Here's how the part is built. I have some questions about the finished solid (model axes, mm). A direction names the side the tool comes from. Give positions to 0.01 mm unless a question says otherwise; leave off trailing zeros. Loops run counter-clockwise (first coordinate to the right, second up) from the corner with the lowest first, then second, coordinate; pieces in that order, holes last. Notation, with made-up numbers: M 7,-28 L 43,-28 A10 cw 43,-13 Z; hole C 21,28.5 d9. An arc over 180 degrees is marked long. Write item = value, one per line. Start each with the question number.
```python
from build123d import *


with BuildPart() as part:
    # Sketch1 → Revolve1 (revolve)
    with BuildSketch(Plane.XY):
        with BuildLine():
            Line((0, 16.845299462), (2, 18))
            Line((2, 18), (10, 18))
            Line((10, 18), (10, 22.5))
            Line((10, 22.5), (37, 22.5))
            ThreePointArc((37, 22.5), (39.121320344, 21.621320344), (40, 19.5))
            Line((40, 19.5), (40, 15))
            Line((40, 15), (12.772080403, 14.049180096))
            ThreePointArc((12.772080403, 14.049180096), (12.22452816, 13.805394131), (12, 13.249667434))
            Line((12, 13.249667434), (12, 5.1))
            Line((12, 5.1), (0, 5.1))
            Line((0, 5.1), (0, 16.845299462))
        make_face()
    revolve(axis=Axis((0, 0, 0), (1, 0, 0)))


solid = part.part
```
Q1. If we section it at D-D, the plane x = 8: List the corners of the cut face in (y, z) for me.
Q2. We'd pull the mould along Y, two halves only. Please class faces 4 (the cylindrical face through (5.9, 2.4, -4.5)), 5 (the flat face through (10, 10.1, 15.1)), 6 (the conical face through (0.13, 16.14, 5.08)): pulls with the +Y half, pulls with the -Y half, needs draft (parallel to the pull), parting line crosses it, or undercut.
Q3. Will these pins go through, and if not, where does the flat tip stop? pin 1 (8 mm diameter, centred on y = 6, z = 2.5, fed in from +X); pin 2 (3 mm diameter, centred on y = 1, z = -1.5, fed in from +X); pin 3 (1 mm diameter, centred on x = 23.5, z = 6.5, fed in from +Y); pin 4 (12 mm diameter, centred on x = 30.5, y = -18, fed in from -Z).
Q4. On a 3-axis mill with a long thin cutter (end or side, diameter ignored), from which of +Z, -Z, +X, -X, +Y, -Y can I reach the whole of each face in a straight line? I mean faces 1 (the flat face through (12, 0, -6)), 2 (the cylindrical face through (6.056, -2.343, 17.847)), 3 (the cylindrical face through (23.689, 10.382, -19.961)). Say none if no direction works.
Q5. If I drill on line 1 along Z through (x, y) = (3, 0); line 2 along Y through (x, z) = (20, -4); line 3 along Y through (x, z) = (2.5, -3), over which ranges is the centre line in solid material (lowest first)?
Q6. If we section it at A-A, the plane z = 0: List the corners of the cut face in (x, y) for me.
Q7. If we section it at C-C, the plane x = 15: List the corners of the cut face in (y, z) for me, then the cut area to 3 significant figures.
Resolved:
q1.outline = C 0,0 d36; hole C 0,0 d10.2
q2.face_4 = undercut
q2.face_5 = needs draft
q2.face_6 = parting line crosses it
q3.pin_1 = 12
q3.pin_2 = through
q3.pin_3 = 21.69
q3.pin_4 = -19.03
q4.face_1 = +X
q4.face_2 = -X
q4.face_3 = +X, -X
q5.line_1 = -18 to -5.1, 5.1 to 18
q5.line_2 = -22.14 to -13.73, 13.73 to 22.14
q5.line_3 = -17.75 to -4.12, 4.12 to 17.75
q6.outline = M 0,-16.85 L 2,-18 L 10,-18 L 10,-22.5 L 37,-22.5 A3 ccw 40,-19.5 L 40,-15 L 12.77,-14.05 A0.8 cw 12,-13.25 L 12,-5.1 L 0,-5.1 Z; M 0,5.1 L 12,5.1 L 12,13.25 A0.8 cw 12.77,14.05 L 40,15 L 40,19.5 A3 ccw 37,22.5 L 10,22.5 L 10,18 L 2,18 L 0,16.85 Z
q7.outline = C 0,0 d45; hole C 0,0 d28.25
q7.area = 963 mm²
